Here's how the part is built. I have some questions about the finished solid (model axes, mm). Face numbers are marked on the shaded views. Coordinates: 2 decimals unless noted, no trailing zeros. Write each loop counter-clockwise with the first axis right and the second up, starting at its lowest first coordinate (ties: lowest second). Pieces come first, ordered by that corner, then holes. Notation, with made-up numbers: (74.25, -35.5) -> (127.25, -35.5) arc R25 cw to (127.25, -6.5) -> close; hole circle Ø5 at (66, 9). An arc over 180 degrees is marked (long way). Use a Markdown table: item, result. Add a question column.
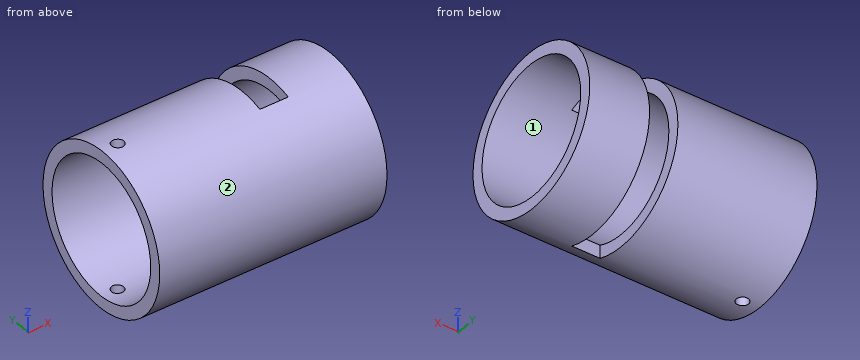
```python
from build123d import *

# Parameters (mm, degrees)
SKETCH1_R               = 25.869040911
SKETCH1_R_2             = 21.869040911
BOSS_EXTRUDE1_DEPTH     = 76
SKETCH2_W               = 9.472494485
SKETCH2_H               = 40.402624636
CUT_EXTRUDE1_DEPTH      = 73.5
CUT_EXTRUDE2_REACH      = 97.509
CUT_EXTRUDE2_END_RADIUS = 21.869040911
SKETCH3_R               = 2
MIRROR1_START           = 21.777395316
MIRROR1_OUTLINE_R       = 2
MIRROR1_DEPTH           = 4.091645695


# Read off the part's stored shape, not the designer's step: Mirror1
with BuildPart() as part:
    # Sketch1 → Boss-Extrude1 (new body)
    with BuildSketch(Plane(origin=(0, 0, 0), x_dir=(0, 0, -1), z_dir=(1, 0, 0))):
        Circle(SKETCH1_R)
        Circle(SKETCH1_R_2, mode=Mode.SUBTRACT)
    extrude(amount=-BOSS_EXTRUDE1_DEPTH)

    # Sketch2 → Cut-Extrude1 (cut, symmetric)
    with BuildSketch(Plane.XY):
        with Locations((-24.754490459, 11.562535947)):
            Rectangle(SKETCH2_W, SKETCH2_H)
    extrude(amount=CUT_EXTRUDE1_DEPTH, both=True, mode=Mode.SUBTRACT)

    # Cut-Extrude2: up to this cylinder (the profile starts outside it)
    cut_extrude2_end = Plane(origin=(-70.565521, 0, 0), z_dir=(1, 0, 0)) * Cylinder(CUT_EXTRUDE2_END_RADIUS, 239.756081822, mode=Mode.PRIVATE)
    # Sketch3 → Cut-Extrude2 (cut, up to the surface)
    with BuildSketch(Plane(origin=(0, 0, -25.869040911), x_dir=(-1, 0, 0), z_dir=(0, 0, -1)), mode=Mode.PRIVATE) as cut_extrude2_sk1:
        with Locations((70.565520642, 0)):
            Circle(SKETCH3_R)
    cut_extrude2_tool1 = extrude(cut_extrude2_sk1.sketch, amount=-CUT_EXTRUDE2_REACH, mode=Mode.PRIVATE) - cut_extrude2_end
    add(cut_extrude2_tool1.solids().sort_by_distance((-70.565521, 0, -25.869041))[0], mode=Mode.SUBTRACT)

    # Mirror1 outline → Mirror1 (cut)
    with BuildSketch(Plane.XY.offset(MIRROR1_START)):
        with Locations((-70.565520642, 0)):
            Circle(MIRROR1_OUTLINE_R)
    extrude(amount=MIRROR1_DEPTH, mode=Mode.SUBTRACT)


solid = part.part
```
Q1. Suppose I cut it at C-C, the plane y = 19. Write out the boundary of the cut face in (x, z), and give its area (3 significant figures).
Q2. Thinking about a two-plate mould opening in Z: for the marked faces 1 and 2, which applies, released by +Z, released by -Z, zero draft, split by the parting line, or undercut?
Q3. Suppose I cut it at B-B, the plane z = 0. Write out the boundary of the cut face in (x, y).
Q4. Suppose I cut it at A-A, the plane y = 0. Write out the boundary of the cut face in (x, z), and give its area (3 significant figures).
Q5. Suppose I cut it at D-D, the plane x = -46. Write out the boundary of the cut face in (y, z).
Q6. Please list where these lines run through material, in increasing order: line 1 (Z direction, x = -39, y = 0); line 2 (Y direction, x = -42.5, z = -19).
Q7. Will these pins go through, and if not, where does the flat tip stop? pin 1 (5 mm diameter, centred on x = -33.5, z = -1, fed in from -Y); pin 2 (1 mm diameter, centred on x = -26.5, y = -19.5, fed in from -Z); pin 3 (3.5 mm diameter, centred on x = -70.57, y = 0, fed in from +Z); pin 4 (1.5 mm diameter, centred on x = -62.5, y = 6.5, fed in from -Z).
Answer key:
| question | item | result |
|---|---|---|
| 1 | outline | (-76, -17.56) -> (-29.49, -17.56) -> (-29.49, -10.83) -> (-76, -10.83) -> close; (-76, 10.83) -> (-29.49, 10.83) -> (-29.49, 17.56) -> (-76, 17.56) -> close; (-20.02, -17.56) -> (0, -17.56) -> (0, -10.83) -> (-20.02, -10.83) -> close; (-20.02, 10.83) -> (0, 10.83) -> (0, 17.56) -> (-20.02, 17.56) -> close |
| 1 | area | 895 mm^2 |
| 2 | face 1 | undercut |
| 2 | face 2 | split by the parting line |
| 3 | outline | (-76, -25.87) -> (0, -25.87) -> (0, -21.87) -> (-76, -21.87) -> close; (-76, 21.87) -> (-29.49, 21.87) -> (-29.49, 25.87) -> (-76, 25.87) -> close; (-20.02, 21.87) -> (0, 21.87) -> (0, 25.87) -> (-20.02, 25.87) -> close |
| 4 | outline | (-76, -25.87) -> (-72.57, -25.87) -> (-72.57, -21.87) -> (-76, -21.87) -> close; (-76, 21.87) -> (-72.57, 21.87) -> (-72.57, 25.87) -> (-76, 25.87) -> close; (-68.57, -25.87) -> (-29.49, -25.87) -> (-29.49, -21.87) -> (-68.57, -21.87) -> close; (-68.57, 21.87) -> (-29.49, 21.87) -> (-29.49, 25.87) -> (-68.57, 25.87) -> close; (-20.02, -25.87) -> (0, -25.87) -> (0, -21.87) -> (-20.02, -21.87) -> close; (-20.02, 21.87) -> (0, 21.87) -> (0, 25.87) -> (-20.02, 25.87) -> close |
| 4 | area | 500 mm^2 |
| 5 | outline | circle Ø51.74 at (0, 0); hole circle Ø43.74 at (0, 0) |
| 6 | line 1 | z = -25.87 to -21.87, 21.87 to 25.87 |
| 6 | line 2 | y = -17.56 to -10.83, 10.83 to 17.56 |
| 7 | pin 1 | stops at y = -25.87 |
| 7 | pin 2 | stops at z = -17.56 |
| 7 | pin 3 | passes through |
| 7 | pin 4 | stops at z = -25.22 |
